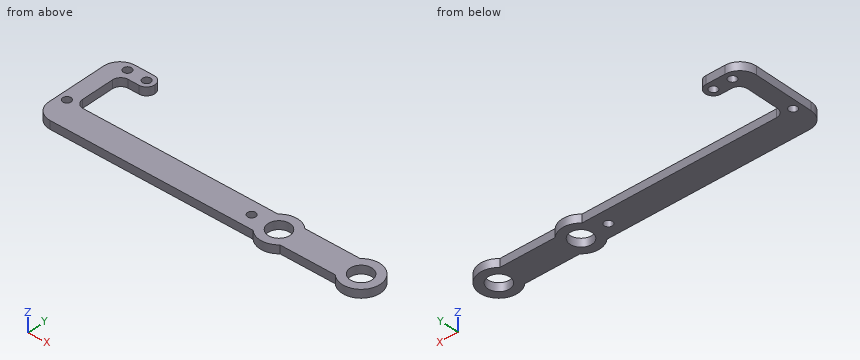
from build123d import *

# Parameters (mm, degrees)
EXTRUDE_1_DEPTH     = 3
CUT_EXTRUDE_START   = -4
SKETCH_3_R          = 4
CUT_EXTRUDE_1_DEPTH = 131.684647847
FILLET_START        = -1
FILLET_1_DEPTH      = 5
FILLET_1_2_DEPTH    = 3
FILLET_2_R          = 6
SKETCH_4_R          = 4
CUT_EXTRUDE_2_DEPTH = 4
SKETCH_5_R          = 1.5
CUT_EXTRUDE_4_DEPTH = 10


with BuildPart() as part:
    # 草图1 → 凸台-拉伸1 (new body)
    with BuildSketch(Plane.XY):
        with BuildLine():
            Line((0, 0), (80.101020514, 0))
            ThreePointArc((80.101020514, 0), (85, -2), (89.898979486, 0))
            Line((89.898979486, 0), (110.101020514, 0))
            ThreePointArc((110.101020514, 0), (122, 5), (110.101020514, 10))
            Line((110.101020514, 10), (89.898979486, 10))
            ThreePointArc((89.898979486, 10), (85, 12), (80.101020514, 10))
            Line((80.101020514, 10), (6, 10))
            Line((6, 10), (6, 28))
            Line((6, 28), (16, 28))
            Line((16, 28), (16, 34))
            Line((16, 34), (0, 34))
            Line((0, 34), (0, 0))
        make_face()
    extrude(amount=EXTRUDE_1_DEPTH)

    # 草图3 → 切除-拉伸1 (cut, through all)
    with BuildSketch(Plane.XY.offset(3).offset(CUT_EXTRUDE_START)):
        with Locations((115, 5)):
            Circle(SKETCH_3_R)
    extrude(amount=CUT_EXTRUDE_1_DEPTH, mode=Mode.SUBTRACT)

    # 圆角1: read off the stored shape, not the designer's step
    # 圆角1 outline → 圆角1 (cut)
    with BuildSketch(Plane.XY.offset(FILLET_START)):
        with BuildLine():
            ThreePointArc((13, 34), (15.121320344, 33.121320344), (16, 31))
            Line((16, 31), (16, 34))
            Line((16, 34), (13, 34))
        make_face()
        with BuildLine():
            ThreePointArc((16, 31), (15.121320344, 28.878679656), (13, 28))
            Line((13, 28), (16, 28))
            Line((16, 28), (16, 31))
        make_face()
    extrude(amount=FILLET_1_DEPTH, mode=Mode.SUBTRACT)

    # Fillet 1 2 outline → Fillet 1 2 (add)
    with BuildSketch(Plane.XY):
        with BuildLine():
            Line((6, 28), (6, 25))
            ThreePointArc((6, 25), (6.878679656, 27.121320344), (9, 28))
            Line((9, 28), (6, 28))
        make_face()
        with BuildLine():
            ThreePointArc((9, 10), (6.878679656, 10.878679656), (6, 13))
            Line((6, 13), (6, 10))
            Line((6, 10), (9, 10))
        make_face()
    extrude(amount=FILLET_1_2_DEPTH)

    # 圆角2
    fillet_2_edges = [part.edges().sort_by_distance(p)[0] for p in [
        (0, 34, 1.5),
        (0, 0, 1.5),
    ]]
    fillet(fillet_2_edges, radius=FILLET_2_R)

    # 草图4 → 切除-拉伸2 (cut)
    with BuildSketch(Plane.XY.offset(3)):
        with Locations((85, 5)):
            Circle(SKETCH_4_R)
    extrude(amount=-CUT_EXTRUDE_2_DEPTH, mode=Mode.SUBTRACT)

    # 草图5 → 切除-拉伸4 (cut)
    with BuildSketch(Plane.XY):
        with Locations((75, 5)):
            Circle(SKETCH_5_R)
        with Locations((3, 10)):
            Circle(SKETCH_5_R)
        with Locations((13, 31)):
            Circle(SKETCH_5_R)
        with Locations((6, 31)):
            Circle(SKETCH_5_R)
    extrude(amount=CUT_EXTRUDE_4_DEPTH, mode=Mode.SUBTRACT)


solid = part.part
Part model, mm, in its own coordinate system. Coordinates: 2 decimals unless noted, no trailing zeros. Order: outer loops, then holes, each group sorted by start corner. A loop starts at its lowest first (then second) coordinate and runs counter-clockwise, first axis right, second up. Notation, with made-up numbers: M 39,-17 L 44,-17 A27 ccw 44,20 Z; hole C -39.5,-5.75 d3. An arc over 180 degrees is marked long. Use a Markdown table: item, result.
(1) Probe L1, parallel to Y at x = 13, z = 1.25; L2, parallel to Y at x = 75, z = 0.6; L3, parallel to X at y = 3, z = 0.8. List the from-to ranges inside material, lowest first.
A:
| item | result |
|---|---|
| L1 | y = 0 to 10, 28 to 29.5, 32.5 to 34 |
| L2 | y = 0 to 3.5, 6.5 to 10 |
| L3 | x = 0.8 to 81.54, 88.46 to 111.54, 118.46 to 121.71 |
(2) Flat gauge pins, fed straight in: pin 1 (1.5 mm diameter, centred on x = 14.5, z = 1, fed in from -Y); pin 2 (0.9 mm diameter, centred on x = 53.5, z = 1.5, fed in from +Y); pin 3 (2.5 mm diameter, centred on x = 75, y = 5, fed in from +Z). Where does each tip first touch, or does it go through?
A:
| item | result |
|---|---|
| pin 1 | stops at y = 0 |
| pin 2 | stops at y = 10 |
| pin 3 | passes through |
(3) Cut at B-B on z = 1.7. Write the cut outline in (x, y), then the cut area to 3 significant figures.
A:
| item | result |
|---|---|
| outline | M 0,6 A6 ccw 6,0 L 80.1,0 A7 ccw 89.9,0 L 110.1,0 A7 ccw long 110.1,10 L 89.9,10 A7 ccw 80.1,10 L 9,10 A3 cw 6,13 L 6,25 A3 cw 9,28 L 13,28 A3 ccw 13,34 L 6,34 A6 ccw 0,28 Z; hole C 3,10 d3; hole C 6,31 d3; hole C 13,31 d3; hole C 75,5 d3; hole C 85,5 d8; hole C 115,5 d8 |
| area | 1,330 mm^2 |
(4) Cut at A-A on x = 75. Write the cut outline in (y, z), then the cut area to 3 significant figures.
A:
| item | result |
|---|---|
| outline | M 0,0 L 3.5,0 L 3.5,3 L 0,3 Z; M 6.5,0 L 10,0 L 10,3 L 6.5,3 Z |
| area | 21.0 mm^2 |
(5) Cut at D-D on y = 21. Write the cut outline in (x, z), then the cut area to 3 significant figures.
A:
| item | result |
|---|---|
| outline | M 0,0 L 6,0 L 6,3 L 0,3 Z |
| area | 18.0 mm^2 |
(6) Cut at C-C on x = 115. Write the cut outline in (y, z), then the cut area to 3 significant figures.
A:
| item | result |
|---|---|
| outline | M -2,0 L 1,0 L 1,3 L -2,3 Z; M 9,0 L 12,0 L 12,3 L 9,3 Z |
| area | 18.0 mm^2 |
